The model under review builds one solid part; all positions refer to its coordinate system, in mm. A direction names the side the tool comes from. Give positions to 0.01 mm unless a question says otherwise; leave off trailing zeros. Order: outer loops, then holes, each group sorted by start corner. A loop starts at its lowest first (then second) coordinate and runs counter-clockwise, first axis right, second up. Notation, with made-up numbers: (-9, 6.25) - (42, 6.25) arc R16 cw to (42, 26.25) - close; hole circle Ø10 at (56.25, 30). An arc over 180 degrees is marked (long way). Write item = value, one per line. Start each with the question number.
1. We need section C-C, the plane x = 6.25. Give the boundary of the cut face in (y, z).
2. We need section B-B, the plane y = 15. Give the boundary of the cut face in (x, z).
3. Wall thickness on probe 1 along X at (y, z) = (28, 0.45); probe 2 along Y at (x, z) = (24, 0.55); probe 3 along Y at (x, z) = (14.5, 0.65): over which ranges is each line inside the solid? List them lowest first.
4. For P1, Ø0.8, axis at y = 6.5, z = 0.5, coming from the -X side; P2, Ø0.8, axis at y = 3.5, z = 0.5, coming from the +X side, all flat-tipped, find the tip position at first contact; note any pin that passes through.
5. Mouldability with a two-part tool opening along Y and no side actions: class faces 6 (the flat face through (1, 0, 1)), 7 (the cylindrical face through (3, 15, 1)), 8 (the flat face through (1.2, 24, 1)), 9 (the flat face through (1.2, 6, 1)) as pulls with the +Y half, pulls with the -Y half, needs draft (parallel to the pull), parting line crosses it, or undercut.
6. We need section A-A, the plane z = 0.5. Give the boundary of the cut face in (x, y), and give its area (3 significant figures).
7. Machinability: for faces 1 (the flat face through (20.712, 41.958, 0.74)), 2 (the flat face through (0, 6, 1)), 3 (the flat face through (3, 31, 1.5)), 4 (the flat face through (26.277, 44.488, 0.74)), 5 (the flat face through (0, 24, 1)), which of the approach directions +Z, -Z, +X, -X, +Y, -Y give a long, thin tool a straight path to every point of the face, cutting with its end or side? Answer none if there is none.
from build123d import *

# Parameters (mm, degrees)
EXTRUDE_THIN1_DEPTH = 1.5
SKETCH2_R           = 3
BOSS_EXTRUDE1_DEPTH = 1.5


with BuildPart() as part:
    # Sketch1 → Extrude-Thin1 (new body)
    with BuildSketch(Plane.XY):
        Polygon((0, 0), (0, 30), (25.980762114, 45), (26.580762114, 43.960769515), (1.2, 29.307179677), (1.2, 0), align=None)
    extrude(amount=EXTRUDE_THIN1_DEPTH)

    # Sketch2 → Boss-Extrude1 (add)
    with BuildSketch(Plane.XY):
        with Locations((12.990381057, 37.5)):
            Circle(SKETCH2_R)
        with Locations((0, 15)):
            Circle(SKETCH2_R)
    extrude(amount=BOSS_EXTRUDE1_DEPTH)


solid = part.part
Model answer:
q1.outline = (32.22, 0) - (33.61, 0) - (33.61, 1.5) - (32.22, 1.5) - close
q2.outline = (-3, 0) - (3, 0) - (3, 1.5) - (-3, 1.5) - close
q3.probe_1 = 0 to 1.2
q3.probe_2 = 42.47 to 43.86
q3.probe_3 = 34.91 to 40.09
q4.P1 = 0
q4.P2 = 1.2
q5.face_6 = pulls with the -Y half
q5.face_7 = undercut
q5.face_8 = undercut
q5.face_9 = needs draft
q6.outline = (0, 0) - (1.2, 0) - (1.2, 12.25) arc R3 ccw to (1.2, 17.75) - (1.2, 29.31) - (11.21, 35.09) arc R3 ccw to (15.97, 37.84) - (26.58, 43.96) - (25.98, 45) - (15.59, 39) arc R3 ccw to (10.39, 36) - (0, 30) - (0, 18) arc R3 ccw to (0, 12) - close
q6.area = 114 mm2
q7.face_1 = +Z, -Z, +Y
q7.face_2 = +Z, -Z, -X, -Y
q7.face_3 = +Z, +X, -X, +Y, -Y
q7.face_4 = +Z, -Z, +X, +Y
q7.face_5 = +Z, -Z, -X, +Y
